from build123d import *

# Parameters (mm, degrees)
F1_DEPTH = 10
F3_DEPTH = 5
F5_DEPTH = 5
F6_R     = 1.5
F7_DEPTH = 2
F8_R     = 1.55
F9_DEPTH = 2.2


with BuildPart() as f1:
    # F0 (on Top) → F1 (new body)
    with BuildSketch(Plane.XY):
        with BuildLine():
            ThreePointArc((-119.543364, -10.458689), (-91.925333, 77.134513), (-10.458689, 119.543364))
            Line((-10.458689, 119.543364), (-10.894468, 124.524337))
            ThreePointArc((-10.894468, 124.524337), (-95.755555, 80.348451), (-124.524337, -10.894468))
            Line((-124.524337, -10.894468), (-119.543364, -10.458689))
        make_face()
    extrude(amount=F1_DEPTH)

    # F2 (on face) → F3 (cut)
    with BuildSketch(Plane(origin=(0, 0, 0), x_dir=(1, 0, 0), z_dir=(0, 0, -1))):
        with BuildLine():
            ThreePointArc((-119.974809, 2.458689), (-119.825869, 6.462291), (-119.543364, 10.458689))
            Line((-119.543364, 10.458689), (-124.524337, 10.894468))
            ThreePointArc((-124.524337, 10.894468), (-124.809525, 6.898011), (-124.966484, 2.894468))
            Line((-124.966484, 2.894468), (-119.974809, 2.458689))
        make_face()
    extrude(amount=-F3_DEPTH, mode=Mode.SUBTRACT)

    # F4 (on face) → F5 (cut)
    with BuildSketch(Plane.XY.offset(10)):
        with BuildLine():
            ThreePointArc((-18.894468, 118.503161), (-14.685791, 119.097975), (-10.458689, 119.543364))
            Line((-10.458689, 119.543364), (-10.894468, 124.524337))
            ThreePointArc((-10.894468, 124.524337), (-14.90221, 124.108518), (-18.894468, 123.563745))
            Line((-18.894468, 123.563745), (-18.894468, 118.503161))
        make_face()
    extrude(amount=-F5_DEPTH, mode=Mode.SUBTRACT)

    # F6 (on face) → F7 (join)
    with BuildSketch(Plane(origin=(0, 0, 5), x_dir=(1, 0, 0), z_dir=(0, 0, -1))):
        with Locations((-122.219087, 6.691388)):
            Circle(F6_R)
    extrude(amount=F7_DEPTH)

    # F8 (on face) → F9 (cut)
    with BuildSketch(Plane.XY.offset(5)):
        with Locations((-14.790966, 121.532989)):
            Circle(F8_R)
    extrude(amount=-F9_DEPTH, mode=Mode.SUBTRACT)


solid = f1.part
Source: CAD feature listing. Evaluate the final solid. Frame: model axes, mm. A direction names the side the tool comes from. Round coordinates to 2 decimals unless told otherwise and drop trailing zeros. Loops run counter-clockwise (first coordinate to the right, second up) from the corner with the lowest first, then second, coordinate; pieces in that order, holes last. Notation, with made-up numbers: M 8,44.25 L 47,44.25 A36 cw 47,78.25 Z; hole C 86.5,13.25 d6. An arc over 180 degrees is marked long. Return JSON: item names as keys, results as strings. Group by question number.
1. Reachability of faces 5 (the face through (-122.51, -2.68, 2.46)), 6 (the face through (-121.53, -5.36, 4.01)), 7 (the face through (-16, 123, 5)), 8 (the face through (-122, -7, 3)) from +Z, -Z, +X, -X, +Y, -Y: full face, straight path, thin tool, end or side. Return the list, or none.
2. Section query A-A on z = 6.75. Output: boundary loops of the cut face in (x, y), and give its area (3 significant figures).
3. Material intervals for line 1 along Y through (x, z) = (-85, 3.25); line 2 along X through (y, z) = (7, 6); line 3 along Y through (x, z) = (-46, 6), sorted ascending. Write a range as from..to.
4. Pin query (flat end, axial travel): pin 1 (5 mm diameter, centred on y = 54, z = 3, fed in from +X); pin 2 (1.8 mm diameter, centred on x = -14.5, y = 121.5, fed in from +Z); pin 3 (5.5 mm diameter, centred on y = 120, z = 8, fed in from +X). Return the tip coordinate at first contact, or that it passes through.
5. Mould query, pull axis X, two halves, no side actions, for faces 1 (the face through (-14.99, 123.07, 3.92)), 2 (the face through (-122.07, -10.68, 7.46)), 3 (the face through (-15, 122, 2.8)), 4 (the face through (-93, 80, 0)). Classes: released by +X, released by -X, zero draft, split by the parting line, or undercut.
6. Section query B-B on x = -57. Output: boundary loops of the cut face in (y, z), and give its area (3 significant figures).
Checks:
{
 "1": {"face 5": "-Z, +X", "face 6": "-Z", "face 7": "+Z, +X, +Y, -Y", "face 8": "-Z, +X, -X, -Y"},
 "2": {"outline": "M -124.52,-10.89 L -119.54,-10.46 A120 cw -18.89,118.5 L -18.89,123.56 A125 ccw Z", "area": "921 mm²"},
 "3": {"line 1": "y = 84.71..91.65", "line 2": "x = -124.8..-119.8", "line 3": "y = 110.83..116.23"},
 "4": {"pin 1": "stops at x = -105.87", "pin 2": "stops at z = 2.8", "pin 3": "stops at x = -18.89"},
 "5": {"face 1": "undercut", "face 2": "released by +X", "face 3": "undercut", "face 4": "zero draft"},
 "6": {"outline": "M 105.6,0 L 111.25,0 L 111.25,10 L 105.6,10 Z", "area": "56.5 mm²"}
}
